```python
from build123d import *

# Parameters (mm, degrees)
CROQUIS1_W              = 10
CROQUIS1_H              = 3
CROQUIS1_W_2            = 3
CROQUIS1_H_2            = 10
CROQUIS1_R              = 5
SALIENTE_EXTRUIR1_DEPTH = 3


with BuildPart() as part:
    # Croquis1 → Saliente-Extruir1 (new body)
    with BuildSketch(Plane.XY):
        Polygon((-35, 71.5), (-45, 71.5), (-45, 68.5), (-55, 68.5), (-55, 71.5), (-65, 71.5), (-65, 68.5), (-72, 68.5), (-72, 61.5), (-75, 61.5), (-75, 51.5), (-72, 51.5), (-72, 41.5), (-75, 41.5), (-75, 31.5), (-72, 31.5), (-72, 21.5), (-75, 21.5), (-75, 11.5), (-72, 11.5), (-72, 1.5), (-75, 1.5), (-75, -8.5), (-72, -8.5), (-72, -18.5), (-75, -18.5), (-75, -28.5), (-72, -28.5), (-72, -38.5), (-75, -38.5), (-75, -48.5), (-72, -48.5), (-72, -51.25), (-65, -51.25), (-65, -54.25), (-72, -54.25), (-72, -58.5), (-75, -58.5), (-75, -68.5), (-72, -68.5), (72, -68.5), (75, -68.5), (75, -58.5), (72, -58.5), (72, -54.25), (65, -54.25), (65, -51.25), (72, -51.25), (72, -48.5), (75, -48.5), (75, -38.5), (72, -38.5), (72, -28.5), (75, -28.5), (75, -18.5), (72, -18.5), (72, -8.5), (75, -8.5), (75, 1.5), (72, 1.5), (72, 11.5), (75, 11.5), (75, 21.5), (72, 21.5), (72, 31.5), (75, 31.5), (75, 41.5), (72, 41.5), (72, 51.5), (75, 51.5), (75, 61.5), (72, 61.5), (72, 68.5), (65, 68.5), (65, 71.5), (55, 71.5), (55, 68.5), (45, 68.5), (45, 71.5), (35, 71.5), (35, 68.5), (25, 68.5), (25, 71.5), (15, 71.5), (15, 68.5), (5, 68.5), (5, 71.5), (-5, 71.5), (-5, 68.5), (-15, 68.5), (-15, 71.5), (-25, 71.5), (-25, 68.5), (-35, 68.5), align=None)
        with Locations((-50, -52.75)):
            Rectangle(CROQUIS1_W, CROQUIS1_H, mode=Mode.SUBTRACT)
        Polygon((-35, -54.25), (-35, -51.25), (-42.5, -51.25), (-42.5, 23.75), (42.5, 23.75), (42.5, -51.25), (35, -51.25), (35, -54.25), (25, -54.25), (25, -51.25), (15, -51.25), (15, -54.25), (5, -54.25), (5, -51.25), (-5, -51.25), (-5, -54.25), (-15, -54.25), (-15, -51.25), (-25, -51.25), (-25, -54.25), align=None, mode=Mode.SUBTRACT)
        with Locations((50, -52.75)):
            Rectangle(CROQUIS1_W, CROQUIS1_H, mode=Mode.SUBTRACT)
        with Locations((50.5, -34.25)):
            Rectangle(CROQUIS1_W_2, CROQUIS1_H_2, mode=Mode.SUBTRACT)
        with Locations((61.473213392, -42.174074015)):
            Circle(CROQUIS1_R, mode=Mode.SUBTRACT)
        with Locations((50.5, -14.25)):
            Rectangle(CROQUIS1_W_2, CROQUIS1_H_2, mode=Mode.SUBTRACT)
        with Locations((-60, 32)):
            Rectangle(CROQUIS1_W, CROQUIS1_H, mode=Mode.SUBTRACT)
        with Locations((-40, 32)):
            Rectangle(CROQUIS1_W, CROQUIS1_H, mode=Mode.SUBTRACT)
        Polygon((-25, 30.5), (-25, 33.5), (-17.5, 33.5), (-17.5, 48.5), (17.5, 48.5), (17.5, 33.5), (25, 33.5), (25, 30.5), (15, 30.5), (15, 33.5), (5, 33.5), (5, 30.5), (-5, 30.5), (-5, 33.5), (-15, 33.5), (-15, 30.5), align=None, mode=Mode.SUBTRACT)
        with Locations((50.5, 5.75)):
            Rectangle(CROQUIS1_W_2, CROQUIS1_H_2, mode=Mode.SUBTRACT)
        with Locations((40, 32)):
            Rectangle(CROQUIS1_W, CROQUIS1_H, mode=Mode.SUBTRACT)
        with Locations((60, 32)):
            Rectangle(CROQUIS1_W, CROQUIS1_H, mode=Mode.SUBTRACT)
    extrude(amount=SALIENTE_EXTRUIR1_DEPTH)


solid = part.part
```
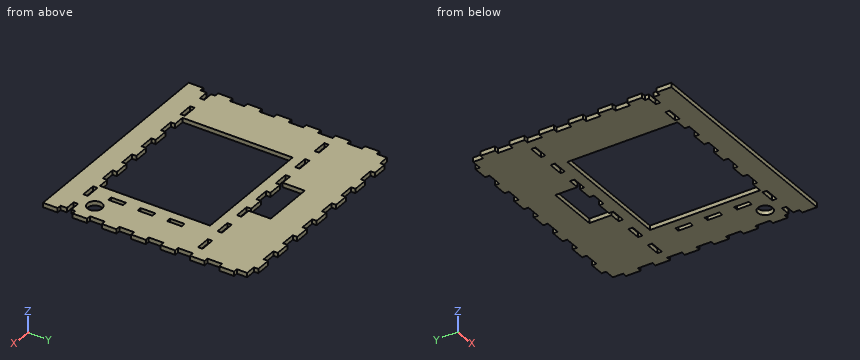
Part model, mm, in its own coordinate system. Round coordinates to 2 decimals unless told otherwise and drop trailing zeros. Order: outer loops, then holes, each group sorted by start corner. A loop starts at its lowest first (then second) coordinate and runs counter-clockwise, first axis right, second up. Notation, with made-up numbers: M -37,44.25 L 9,44.25 A37 cw 9,80.25 Z; hole C 9.25,87 d10. An arc over 180 degrees is marked long. Put each result on its own line as item: value. Start each with the question number.
1. Drill centre lines: probe 1 along X at (y, z) = (-31, 1.8); probe 2 along Y at (x, z) = (24, 2.4); probe 3 along Y at (x, z) = (30.5, 2.3). Where is each one in solid material? Low to high. Write a range as [from, to].
2. Slice it at D-D on y = 9. List the corners of the cut face in (x, z), then the cut area to 3 significant figures.
3. Slice it at C-C on x = -12.5. List the corners of the cut face in (y, z), then the cut area to 3 significant figures.
4. Drop flat-ended pins along their axis: pin 1 (1.5 mm diameter, centred on y = -52.5, z = 2, fed in from +X); pin 2 (1.5 mm diameter, centred on x = 67, z = 1, fed in from +Y); pin 3 (1.5 mm diameter, centred on y = 44, z = 0.5, fed in from -X). Give the stop position or say it passes through.
5. Slice it at A-A on x = -31.5. List the corners of the cut face in (y, z).
6. Slice it at B-B on y = 37. List the corners of the cut face in (x, z), then the cut area to 3 significant figures.
Findings:
1. probe 1: [-72, -42.5], [42.5, 49], [52, 72]
1. probe 2: [-68.5, -51.25], [23.75, 30.5], [33.5, 71.5]
1. probe 3: [-68.5, -54.25], [23.75, 68.5]
2. outline: M -72,0 L -42.5,0 L -42.5,3 L -72,3 Z; M 42.5,0 L 49,0 L 49,3 L 42.5,3 Z; M 52,0 L 72,0 L 72,3 L 52,3 Z
2. area: 168 mm2
3. outline: M -68.5,0 L -54.25,0 L -54.25,3 L -68.5,3 Z; M 23.75,0 L 33.5,0 L 33.5,3 L 23.75,3 Z; M 48.5,0 L 68.5,0 L 68.5,3 L 48.5,3 Z
3. area: 132 mm2
4. pin 1: x = 65
4. pin 2: y = 68.5
4. pin 3: x = -72
5. outline: M -68.5,0 L -54.25,0 L -54.25,3 L -68.5,3 Z; M 23.75,0 L 68.5,0 L 68.5,3 L 23.75,3 Z
6. outline: M -75,0 L -17.5,0 L -17.5,3 L -75,3 Z; M 17.5,0 L 75,0 L 75,3 L 17.5,3 Z
6. area: 345 mm2
